Verification items for the finished model (mm, model axes). A direction names the side the tool comes from. Coordinates: 2 decimals unless noted, no trailing zeros. Order: outer loops, then holes, each group sorted by start corner. A loop starts at its lowest first (then second) coordinate and runs counter-clockwise, first axis right, second up. Notation, with made-up numbers: M 45.5,67.5 L 103.5,67.5 A23 cw 103.5,90.5 Z; hole C 20,1 d4. An arc over 180 degrees is marked long. Return JSON: item names as keys, results as strings. Group by question number.
1. Section check D-D, the plane x = 17. Record the cut outline in (y, z) (1 decimal), plus the area to 3 significant figures.
2. Material ranges on line 1 along X through (y, z) = (158, -17.5) (3 decimals); line 2 along Z through (x, y) = (-30, 156.5), recorded low to high.
3. Set-up check for faces 1 (the flat face through (-14, -188.912, -31)), 2 (the flat face through (5, -3, -28.575)): record each of +Z, -Z, +X, -X, +Y, -Y from which the full face is reachable in a straight line by a thin tool's end or side.
4. Gauge pin test, flat ends, axial feed: pin 1 (8.5 mm diameter, centred on y = -98.425, z = 0, fed in from -X); pin 2 (5 mm diameter, centred on y = -87, z = -30.5, fed in from +X); pin 3 (2 mm diameter, centred on y = 56, z = 29, fed in from +X) (3 decimals); pin 4 (12 mm diameter, centred on x = -17.5, y = 47.5, fed in from +Z) (3 decimals). Record the tip position at first contact, or that the pin passes through.
5. Section check C-C, the plane y = -62. Record the cut outline in (x, z) (3 decimals), plus the area to 3 significant figures.
6. Section check A-A, the plane z = 0. Record the cut outline in (x, y) (1 decimal), plus the area to 3 significant figures.
7. Section check B-B, the plane y = -102. Record the cut outline in (x, z) (3 decimals).
```python
from build123d import *

# Parameters (mm, degrees)
F1_DEPTH = 188.9125
F2_R     = 5.08
F3_R     = 7.14375
F4_DEPTH = 25.4


with BuildPart() as f1:
    # F0 (on Front) → F1 (new body, symmetric)
    with BuildSketch(Plane.XZ):
        Polygon((-38.1, -38.1), (38.1, -38.1), (38.1, -28.575), (-28.575, -28.575), (-28.575, 38.1), (-38.1, 38.1), align=None)
    extrude(amount=F1_DEPTH, both=True)

    # F2
    f2_edges = [f1.edges().sort_by_distance(p)[0] for p in [
        (-28.575, 0, 38.1),
        (-28.575, 0, -28.575),
        (38.1, 0, -28.575),
    ]]
    fillet(f2_edges, radius=F2_R)

    # F3 (on face) → F4 (cut)
    with BuildSketch(Plane(origin=(-38.1, 0, 0), x_dir=(0, -1, 0), z_dir=(-1, 0, 0))):
        with Locations((-98.425, 0)):
            Circle(F3_R)
        with Locations((98.425, 0)):
            Circle(F3_R)
    extrude(amount=-F4_DEPTH, mode=Mode.SUBTRACT)


solid = f1.part
```
Answers follow:
{
 "1": {"outline": "M -188.9,-38.1 L 188.9,-38.1 L 188.9,-28.6 L -188.9,-28.6 Z", "area": "3,600 mm^2"},
 "2": {"line 1": "-38.1 to -28.575", "line 2": "-38.1 to 36.55"},
 "3": {"face 1": "+Z, -Z, +X, -X, -Y", "face 2": "+Z, +X, +Y, -Y"},
 "4": {"pin 1": "through", "pin 2": "x = 38.06", "pin 3": "x = -28.575", "pin 4": "z = -28.575"},
 "5": {"outline": "M -38.1,-38.1 L 38.1,-38.1 L 38.1,-33.655 A5.08 ccw 33.02,-28.575 L -23.495,-28.575 A5.08 cw -28.575,-23.495 L -28.575,33.02 A5.08 ccw -33.655,38.1 L -38.1,38.1 Z", "area": "1,360 mm^2"},
 "6": {"outline": "M -38.1,-188.9 L -28.6,-188.9 L -28.6,-105.6 L -38.1,-105.6 Z; M -38.1,-91.3 L -28.6,-91.3 L -28.6,91.3 L -38.1,91.3 Z; M -38.1,105.6 L -28.6,105.6 L -28.6,188.9 L -38.1,188.9 Z", "area": "3,330 mm^2"},
 "7": {"outline": "M -38.1,-38.1 L 38.1,-38.1 L 38.1,-33.655 A5.08 ccw 33.02,-28.575 L -23.495,-28.575 A5.08 cw -28.575,-23.495 L -28.575,-6.185 L -38.1,-6.185 Z; M -38.1,6.185 L -28.575,6.185 L -28.575,33.02 A5.08 ccw -33.655,38.1 L -38.1,38.1 Z"}
}
